Input: part model. Units: mm. Frame: model coordinates. Face numbers are marked on the shaded views. A direction names the side the tool comes from. Give positions to 0.01 mm unless a question says otherwise; leave off trailing zeros. Write each loop counter-clockwise with the first axis right and the second up, starting at its lowest first coordinate (ties: lowest second). Pieces come first, ordered by that corner, then holes.
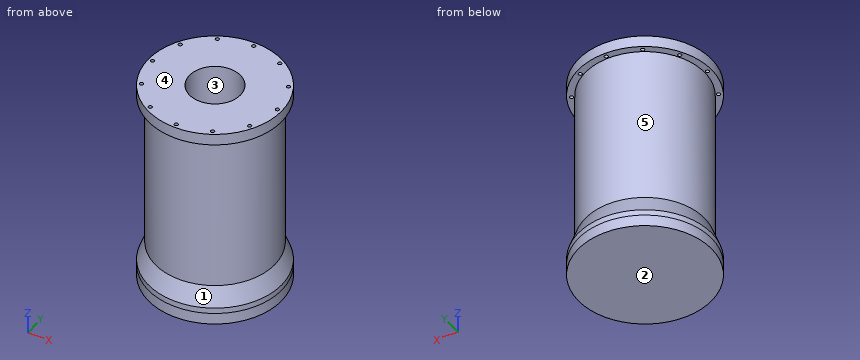
```python
from build123d import *

# Parameters (mm, degrees)
SKETCH2_R           = 73.66
BOSS_EXTRUDE1_DEPTH = 12.7
SKETCH3_R           = 66
BOSS_EXTRUDE2_DEPTH = 203.2
SKETCH4_R           = 73.66
BOSS_EXTRUDE3_DEPTH = 12.7
SKETCH6_R           = 2
CUT_EXTRUDE1_DEPTH  = 12.7
CHAMFER1_SIZE       = 27.474774195
CHAMFER1_SIZE_2     = 10
SKETCH8_R           = 28.1625529
CUT_EXTRUDE2_DEPTH  = 150


with BuildPart() as part:
    # Sketch2 → Boss-Extrude1 (new body)
    with BuildSketch(Plane.XY):
        Circle(SKETCH2_R)
    extrude(amount=BOSS_EXTRUDE1_DEPTH)

    # Sketch3 → Boss-Extrude2 (add)
    with BuildSketch(Plane.XY.offset(12.7)):
        Circle(SKETCH3_R)
    extrude(amount=BOSS_EXTRUDE2_DEPTH)

    # Sketch4 → Boss-Extrude3 (add)
    with BuildSketch(Plane.XY.offset(215.9)):
        Circle(SKETCH4_R)
    extrude(amount=BOSS_EXTRUDE3_DEPTH)

    # Sketch6 → Cut-Extrude1 (cut)
    with BuildSketch(Plane.XY.offset(228.6)):
        with Locations((0, 69)):
            Circle(SKETCH6_R)
        with Locations((34.5, 59.755752861)):
            Circle(SKETCH6_R)
        with Locations((59.755752861, 34.5)):
            Circle(SKETCH6_R)
        with Locations((69, 0)):
            Circle(SKETCH6_R)
        with Locations((59.755752861, -34.5)):
            Circle(SKETCH6_R)
        with Locations((34.5, -59.755752861)):
            Circle(SKETCH6_R)
        with Locations((0, -69)):
            Circle(SKETCH6_R)
        with Locations((-34.5, -59.755752861)):
            Circle(SKETCH6_R)
        with Locations((-59.755752861, -34.5)):
            Circle(SKETCH6_R)
        with Locations((-69, 0)):
            Circle(SKETCH6_R)
        with Locations((-59.755752861, 34.5)):
            Circle(SKETCH6_R)
        with Locations((-34.5, 59.755752861)):
            Circle(SKETCH6_R)
    extrude(amount=-CUT_EXTRUDE1_DEPTH, mode=Mode.SUBTRACT)

    # Chamfer1
    # the kernel refuses this chamfer: 27.474774195, 10 mm, written as the material it adds along each edge
    with BuildSketch(Plane(origin=(0, 0, 12.7), x_dir=(1, 0, 0), z_dir=(0, -1, 0))) as chamfer1_piece_1_section:
        Polygon((66, CHAMFER1_SIZE), (66 + CHAMFER1_SIZE_2, 0), (66, 0), align=None)
    chamfer1_piece_1 = revolve(axis=Axis((0, 0, 12.7), (0, 0, 1)), mode=Mode.PRIVATE)
    chamfer1_piece_1 = chamfer1_piece_1 & Plane(origin=(0, 0, 30.030529596), x_dir=(1, 0, 0), z_dir=(0, 0, -1)) * Cylinder(73.66, 304, mode=Mode.PRIVATE)
    add(chamfer1_piece_1)

    # Sketch8 → Cut-Extrude2 (cut)
    with BuildSketch(Plane.XY.offset(228.6)):
        Circle(SKETCH8_R)
    extrude(amount=-CUT_EXTRUDE2_DEPTH, mode=Mode.SUBTRACT)


solid = part.part
```
Item 1: Ray query, line 1 (Y direction, x = 0, z = 223.25); line 2 (Y direction, x = 34, z = 221); line 3 (Y direction, x = 0, z = 131.5). Return the intervals inside material, ascending.
Item 2: Pin query (flat end, axial travel): pin 1 (8 mm diameter, centred on x = -7, z = 184.5, fed in from +Y); pin 2 (8 mm diameter, centred on x = -27, z = 61.5, fed in from -Y); pin 3 (1.5 mm diameter, centred on y = 48.5, z = 65, fed in from -X). Return the tip coordinate at first contact, or that it passes through.
Item 3: Section B-B (z = 36.5). Return loops of the section in (x, y).
Item 4: Set-up query: the marked faces 4 and 5. Return all of +Z, -Z, +X, -X, +Y, -Y with unobstructed straight access to the full face (end or side cutting, diameter ignored); none if empty.
Item 5: Mould query, pull axis Z, two halves, no side actions, for the marked faces 1, 2 and 3. Classes: +Z half, -Z half, draft (parallel to the pull), parting line (faces both ways), or undercut.
Item 6: Section A-A (z = 207.5). Return loops of the section in (x, y), and give its area (3 significant figures).
Solved:
1. line 1: y = -73.66 to -71, -67 to -28.16, 28.16 to 67, 71 to 73.66
1. line 2: y = -65.34 to -61.69, -57.82 to 57.82, 61.69 to 65.34
1. line 3: y = -66 to -28.16, 28.16 to 66
2. pin 1: stops at y = 65.93
2. pin 2: stops at y = -61.86
2. pin 3: stops at x = -45.56
3. outline: circle Ø134.68 at (0, 0)
4. face 4: +Z, +X, -X, +Y, -Y
4. face 5: none
5. face 1: undercut
5. face 2: -Z half
5. face 3: draft
6. outline: circle Ø132 at (0, 0); hole circle Ø56.33 at (0, 0)
6. area: 11,200 mm2
